Work out the finished part from the listing and answer in its coordinate system (mm). Face numbers are marked on the shaded views. A direction names the side the tool comes from. Give positions to 0.01 mm unless a question says otherwise; leave off trailing zeros. Loops run counter-clockwise (first coordinate to the right, second up) from the corner with the lowest first, then second, coordinate; pieces in that order, holes last. Notation, with made-up numbers: (28, 75.25) - (46, 75.25) arc R8 ccw to (46, 86.25) - close; hole circle Ø2 at (34.25, 56.25). An arc over 180 degrees is marked (long way). One line per item, written item: value.
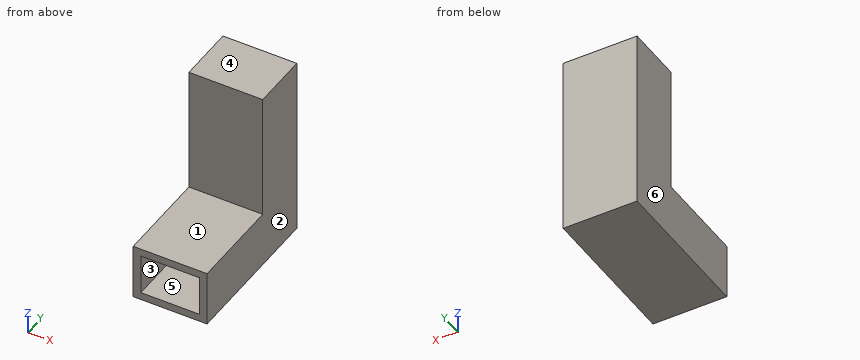
from build123d import *

# Parameters (mm, degrees)
EXTRUDE_1_DEPTH     = 9.7
SKETCH_2_W          = 7.7
SKETCH_2_H          = 5.316419403
CUT_EXTRUDE_1_DEPTH = 17


with BuildPart() as part:
    # 草圖1 → 填料-伸長1 (new body)
    with BuildSketch(Plane(origin=(0, 0, 0), x_dir=(0, 0, -1), z_dir=(1, 0, 0))):
        Polygon((0, 0), (0, 20), (-24, 20), (-24, 12.4126021), (-7.316419403, 12.4126021), (-7.316419403, 0), align=None)
    extrude(amount=EXTRUDE_1_DEPTH)

    # 草圖2 → 除料-伸長1 (cut)
    with BuildSketch(Plane.XZ):
        with Locations((4.85, 3.658209702)):
            Rectangle(SKETCH_2_W, SKETCH_2_H)
    extrude(amount=-CUT_EXTRUDE_1_DEPTH, mode=Mode.SUBTRACT)


solid = part.part
1. Flat-ended cylindrical pins translate along their axes: pin 1 Ø3 at (x, z) = (6.5, 19.5) entering from -Y; pin 2 Ø2.5 at (x, z) = (4.5, 3.5) entering from -Y; pin 3 Ø1.5 at (y, z) = (8, 9) entering from -X; pin 4 Ø3 at (x, y) = (5.5, 4.5) entering from +Z. Find the tip coordinate at first contact, or state that the pin passes through.
Output:
pin 1: stops at y = 12.41
pin 2: stops at y = 17
pin 3: passes through
pin 4: stops at z = 7.32
2. For the marked faces 1, 2 and 3, determine the directions among +Z, -Z, +X, -X, +Y, -Y from which every point of the face is accessible in a straight line to the end or side of a thin tool.
Output:
face 1: +Z, +X, -X, -Y
face 2: +Z, -Z, +X, +Y, -Y
face 3: -Y
3. Section C-C (x = 4.5) is taken. Write down the section's boundary in (y, z), and give its area (3 significant figures).
Output:
outline: (0, 0) - (20, 0) - (20, 24) - (12.41, 24) - (12.41, 7.32) - (0, 7.32) - (0, 6.32) - (17, 6.32) - (17, 1) - (0, 1) - close
area: 183 mm²
4. Section B-B (z = 4.5) is taken. Write down the section's boundary in (x, y).
Output:
outline: (0, 0) - (1, 0) - (1, 17) - (8.7, 17) - (8.7, 0) - (9.7, 0) - (9.7, 20) - (0, 20) - close
5. Section A-A (y = 13) is taken. Write down the section's boundary in (x, z), and give its area (3 significant figures).
Output:
outline: (0, 0) - (9.7, 0) - (9.7, 24) - (0, 24) - close; hole (1, 1) - (8.7, 1) - (8.7, 6.32) - (1, 6.32) - close
area: 192 mm²
6. The mould has two halves that part along Z. Classify the marked faces 4, 5 and 6: released by +Z, released by -Z, zero draft, split by the parting line, or undercut.
Output:
face 4: released by +Z
face 5: undercut
face 6: zero draft
7. Find the intervals of material crossed by line 1 along X through (y, z) = (10.5, 3); line 2 along Z through (x, y) = (1.25, 15); line 3 along Z through (x, y) = (6.75, 6.5), in increasing order.
Output:
line 1: x = 0 to 1, 8.7 to 9.7
line 2: z = 0 to 1, 6.32 to 24
line 3: z = 0 to 1, 6.32 to 7.32
8. Section D-D (y = 11) is taken. Write down the section's boundary in (x, z).
Output:
outline: (0, 0) - (9.7, 0) - (9.7, 7.32) - (0, 7.32) - close; hole (1, 1) - (8.7, 1) - (8.7, 6.32) - (1, 6.32) - close
